Autodesk Inventor part; units mm, degrees
ref_plane "YZ Plane" through (0, 0, 0) normal (1, 0, 0) x (0, 1, 0)
ref_plane "XZ Plane" through (0, 0, 0) normal (0, 1, 0) x (-1, 0, 0)
ref_plane "XY Plane" through (0, 0, 0) normal (0, 0, 1) x (1, 0, 0)
sketch "スケッチ1" plane through (0, 0, 0) normal (0, 0, 1) x (1, 0, 0)
  line L0 (-59, -17.25) -> (53, -17.25) construction
  line L1 (1.6, -41.5) -> (-1.6, -41.5) construction
  line L2 (-1.6, -41.5) -> (-1.6, -43.5)
  line L3 (-1.6, -43.5) -> (1.6, -43.5) construction
  line L4 (1.6, -43.5) -> (1.6, -41.5)
  arc A0 (1.6, -41.5) -> (-1.6, -41.5) centre (0, -41.5) ccw
  arc A1 (-1.6, -43.5) -> (1.6, -43.5) centre (0, -43.5) ccw
  circle A2 centre (0, -42.5) radius 1.5 construction
  line L5 (0, -41.5) -> (0, -42.5) construction
  line L6 (0, -42.5) -> (0, -43.5) construction
  line L7 (0, -41.5) -> (0, -17.25) construction
  line L8 (0, -17.25) -> (-20, -17.25)
  line L9 (-20, -17.25) -> (-20, -21.25)
  line L10 (0, -17.25) -> (20, -17.25)
  line L11 (20, -17.25) -> (20, -21.25)
  arc A3 (-3.7095, -44.9966) -> (3.7095, -44.9966) centre (0, -43.5) ccw
  arc A4 (-3.7095, -44.9966) -> (-19.3339, -22.7402) centre (-59.3515, -67.4458) ccw
  arc A5 (19.3339, -22.7402) -> (3.7095, -44.9966) centre (59.3515, -67.4458) ccw
  arc A6 (-20, -21.25) -> (-19.3339, -22.7402) centre (-18, -21.25) ccw
  arc A7 (19.3339, -22.7402) -> (20, -21.25) centre (18, -21.25) ccw
  arc A8 (-3.2471, -36.6513) -> (-10.9625, -25.559) centre (-59.3515, -67.4458) ccw
  arc A9 (10.9625, -25.559) -> (3.2471, -36.6513) centre (59.3515, -67.4458) ccw
  arc A10 (0.9959, -37.626) -> (-0.9959, -37.626) centre (0, -41.5) ccw
  line L12 (-9.4504, -22.25) -> (9.4504, -22.25)
  arc A11 (-9.4504, -22.25) -> (-10.9625, -25.559) centre (-9.4504, -24.25) ccw
  arc A12 (10.9625, -25.559) -> (9.4504, -22.25) centre (9.4504, -24.25) ccw
  arc A13 (0.9959, -37.626) -> (3.2471, -36.6513) centre (1.4939, -35.6889) ccw
  arc A14 (-3.2471, -36.6513) -> (-0.9959, -37.626) centre (-1.4939, -35.6889) ccw
  point P0 (0, 0)
  point P1 (-20, -22.1528)
  point P2 (20, -22.1528)
  dimension "d0" = 2
  dimension "d1" = 1.6
  dimension "d3" = 4
  dimension "d4" = 2
  dimension "d5" = 4
  dimension "d6" = 60
  dimension "d7" = 20
  dimension "d8" = 4
  dimension "d9" = 4
  dimension "d10" = 2.4
  dimension "d11" = 5
  dimension "d12" = 2
extrude "押し出し1" add sketch "スケッチ1" against normal blind 1.5
sketch "スケッチ2" plane through (-20, -17.25, 0) normal (0, 1, 0) x (1, 0, 0)
  line L0 (40, 0) -> (0, 0) construction
  line L1 (40, 0) -> (0, 0)
  line L2 (0, 0) -> (0, -4.5)
  line L3 (0.5, -5) -> (3, -5)
  line L4 (40, -4.5) -> (40, 0)
  line L5 (0, 0) -> (0, 1.5) construction
  line L6 (69.5, -5) -> (-3.5, -5) construction
  line L7 (20, 0) -> (20, -8.2375) construction
  circle A0 centre (35.5, -3) radius 1.1
  line L8 (40, -4.5) -> (39.5, -5)
  line L9 (0.5, -5) -> (0, -4.5)
  arc A1 (34, -5) -> (37, -5) centre (35.5, -3) ccw
  line L10 (37, -5) -> (39.5, -5)
  line L11 (34, -5) -> (37, -5) construction
  circle A2 centre (4.5, -3) radius 1.1
  arc A3 (3, -5) -> (6, -5) centre (4.5, -3) ccw
  line L12 (6, -5) -> (34, -5)
  line L13 (3, -5) -> (6, -5) construction
  point P0 (40, -5)
  point P1 (0, -5)
  dimension "d18" = 2.2
  dimension "d19" = 0.5
  dimension "d20" = 0.5
  dimension "d21" = 0.5
  dimension "d22" = 0.5
  dimension "d23" = 2.5
  dimension "d24" = 4.5
  dimension "d25" = 2
extrude "押し出し2" add sketch "スケッチ2" against normal blind 1.5
properties part number "NUC_tab"
Geometry check sheet. Reference: the model listing, model coordinates, mm. A direction names the side the tool comes from. Coordinates: 2 decimals unless noted, no trailing zeros. Loops run counter-clockwise (first coordinate to the right, second up) from the corner with the lowest first, then second, coordinate; pieces in that order, holes last. Notation, with made-up numbers: (4.5, 0) -> (32.5, 0) arc R15 cw to (32.5, 26) -> close; hole circle Ø2 at (-13, -17). An arc over 180 degrees is marked (long way). Put each result on its own line as item: value.
1) Cross-section at B-B on y = -24.5. Record the boundary of the cut face in (x, z), plus the area to 3 significant figures.
Result set:
outline: (-17.45, -1.5) -> (-11.43, -1.5) -> (-11.43, 0) -> (-17.45, 0) -> close; (11.43, -1.5) -> (17.45, -1.5) -> (17.45, 0) -> (11.43, 0) -> close
area: 18.0 mm^2
2) Gauge pin test, flat ends, axial feed: pin 1 Ø1.2 at (x, y) = (18, -18) entering from +Z; pin 2 Ø12 at (x, y) = (-11, -44) entering from -Z; pin 3 Ø0.8 at (y, z) = (-42.5, -1) entering from -X; pin 4 Ø3 at (x, z) = (3.5, 3.5) entering from -Y. Record the tip position at first contact, or that the pin passes through.
Result set:
pin 1: stops at z = 5
pin 2: passes through
pin 3: stops at x = -4.97
pin 4: stops at y = -18.75
3) Tool access check on faces 5 (the cylindrical face through (11.283, -23.448, -0.74)), 6 (the flat face through (-18, -18, 5)), 7 (the flat face through (1, -21, 0)). Record the directions out of +Z, -Z, +X, -X, +Y, -Y that give a thin tool (end or side, any length) a straight path to the whole face; none if there is none.
Result set:
face 5: +Z, -Z
face 6: +Z, -X, +Y, -Y
face 7: +Z, +X, -X, -Y
4) Cross-section at D-D on z = 3.5. Record the boundary of the cut face in (x, y).
Result set:
outline: (-20, -18.75) -> (-16.48, -18.75) -> (-16.48, -17.25) -> (-20, -17.25) -> close; (-14.52, -18.75) -> (14.52, -18.75) -> (14.52, -17.25) -> (-14.52, -17.25) -> close; (16.48, -18.75) -> (20, -18.75) -> (20, -17.25) -> (16.48, -17.25) -> close
5) Cross-section at C-C on x = 15.5. Record the boundary of the cut face in (y, z), plus the area to 3 significant figures.
Result set:
outline: (-26.49, -1.5) -> (-17.25, -1.5) -> (-17.25, 1.9) -> (-18.75, 1.9) -> (-18.75, 0) -> (-26.49, 0) -> close; (-18.75, 4.1) -> (-17.25, 4.1) -> (-17.25, 5.5) -> (-18.75, 5.5) -> close
area: 18.8 mm^2
6) Cross-section at A-A on x = 0. Record the boundary of the cut face in (y, z), plus the area to 3 significant figures.
Result set:
outline: (-47.5, -1.5) -> (-45.1, -1.5) -> (-45.1, 0) -> (-47.5, 0) -> close; (-39.9, -1.5) -> (-37.5, -1.5) -> (-37.5, 0) -> (-39.9, 0) -> close; (-22.25, -1.5) -> (-17.25, -1.5) -> (-17.25, 5) -> (-18.75, 5) -> (-18.75, 0) -> (-22.25, 0) -> close
area: 22.2 mm^2
7) Thickness scan on line 1 (X direction, y = -17.55, z = 3); line 2 (Z direction, x = -15.5, y = -17.8); line 3 (Z direction, x = 13, y = -28). Record the ranges inside material, lowest first.
Result set:
line 1: x = -20 to -16.6, -14.4 to 14.4, 16.6 to 20
line 2: z = -1.5 to 1.9, 4.1 to 5.5
line 3: z = -1.5 to 0
8) Release check for a two-part mould opening along Y. For faces 1 (the flat face through (0, -22.25, -1)), 2 (the flat face through (1.6, -43, -1)), 3 (the cylindrical face through (-15.5, -18, 5.5)), 4 (the cylindrical face through (10.355, -32.815, -0.74)) record: released by +Y, released by -Y, zero draft, split by the parting line, or undercut.
Result set:
face 1: undercut
face 2: undercut
face 3: zero draft
face 4: released by -Y
